Input: part model. Units: mm. Frame: model coordinates. A direction names the side the tool comes from. Give positions to 0.01 mm unless a question says otherwise; leave off trailing zeros. Loops run counter-clockwise (first coordinate to the right, second up) from the corner with the lowest first, then second, coordinate; pieces in that order, holes last. Notation, with made-up numbers: M -8.5,78 L 28.5,78 A31 cw 28.5,107 Z; hole C -11.5,89.5 d7. An arc over 180 degrees is marked long. Answer as a JSON object with one key per item and string values. Group by question number.
1) Section query C-C on y = 14.5. Return loops of the section in (x, z), plus the area to 3 significant figures.
2) Section query D-D on z = 1.5. Return loops of the section in (x, y).
3) Ray query, L1, parallel to X at y = 0, z = 8.5; L2, parallel to Y at x = 0, z = 9.25; L3, parallel to Y at x = -1, z = 3. Return the intervals inside material, ascending.
4) First-contact query: P1, Ø12, axis at y = 23, z = 7, coming from the -X side; P2, Ø8, axis at y = 26.5, z = 13.5, coming from the +X side; P3, Ø2.5, axis at x = -0.5, z = 5, coming from the +Y side; P4, Ø5, axis at x = 0.5, z = 17, coming from the -Y side. Flat tips, straight axial feed; report the tip coordinate or a pass-through.
5) Access query for faces 1 (the flat face through (-1.877, 3.143, 9.86)), 2 (the flat face through (-2.5, 24, 10)), 3 (the flat face through (0, 3.921, 5)), 4 (the flat face through (0, 43.921, 9.6)). Directions: +Z, -Z, +X, -X, +Y, -Y. A direction counts if a zero-diameter tool reaches every point of the face in a straight line with its end or side. Return the directions, or none.
6) Draft query along Z for faces 5 (the flat face through (2.5, 24, 10)), 6 (the cylindrical face through (-0.04, 40.91, 17.15)), 7 (the flat face through (0, 5, 2.5)). Return one class per face: +Z half, -Z half, draft (parallel to the pull), parting line (faces both ways), or undercut.
7) Section query B-B on z = 15. Return loops of the section in (x, y), plus the area to 3 significant figures.
8) Section query A-A on x = 1. Return loops of the section in (y, z).
from build123d import *

# Parameters (mm, degrees)
F1_DEPTH = 20
F3_DEPTH = 7.151
F4_R     = 10
F5_SIZE  = 5
F6_R     = 10


with BuildPart() as f1:
    # F0 (on Top) → F1 (new body)
    with BuildSketch(Plane.XY):
        with BuildLine():
            ThreePointArc((2.65, 0), (-0.9156644986, -2.4867767343), (-2.0172139819, 1.7185306955))
            Line((-2.0172139819, 1.7185306955), (-2.6488466474, 2.5070635361))
            Line((-2.6488466474, 2.5070635361), (-3.2804793129, 3.2955963767))
            ThreePointArc((-3.2804793129, 3.2955963767), (-1.7844146372, -4.2939916631), (4.65, 0))
            ThreePointArc((4.65, 0), (4.0772233199, 2.2357884515), (2.5, 3.920777984))
            ThreePointArc((2.5, 3.920777984), (1.3020910825, 4.4639734333), (0, 4.65))
            Line((0, 4.65), (0, 2.65))
            ThreePointArc((0, 2.65), (1.8738329701, 1.8738329701), (2.65, 0))
        make_face()
        with BuildLine():
            Line((0, 43.920777984), (0, 4.65))
            ThreePointArc((0, 4.65), (1.3020910825, 4.4639734333), (2.5, 3.920777984))
            Line((2.5, 3.920777984), (2.5, 43.920777984))
            Line((2.5, 43.920777984), (0, 43.920777984))
        make_face()
        with BuildLine():
            ThreePointArc((-1.236734669, 2.3437123028), (-0.6370488198, 2.572288631), (0, 2.65))
            Line((0, 2.65), (0, 4.65))
            ThreePointArc((0, 4.65), (-1.3020910825, 4.4639734333), (-2.5, 3.920777984))
            Line((-2.5, 3.920777984), (-1.8683673345, 3.1322451434))
            Line((-1.8683673345, 3.1322451434), (-1.236734669, 2.3437123028))
        make_face()
        with BuildLine():
            ThreePointArc((-2.5, 3.920777984), (-1.3020910825, 4.4639734333), (0, 4.65))
            Line((0, 4.65), (0, 43.920777984))
            Line((0, 43.920777984), (-2.5, 43.920777984))
            Line((-2.5, 43.920777984), (-2.5, 3.920777984))
        make_face()
    extrude(amount=F1_DEPTH)

    # F2 (on face) → F3 (cut, through all)
    with BuildSketch(Plane(origin=(-2.5, 0, 0), x_dir=(0, -1, 0), z_dir=(-1, 0, 0))):
        with BuildLine():
            Line((-33.920777984, 10), (-33.920777984, 12.25))
            ThreePointArc((-33.920777984, 12.25), (-35.5117682417, 11.5909902577), (-36.170777984, 10))
            Line((-36.170777984, 10), (-33.920777984, 10))
        make_face()
        with BuildLine():
            ThreePointArc((-36.170777984, 10), (-33.920777984, 7.75), (-31.670777984, 10))
            ThreePointArc((-31.670777984, 10), (-32.3297877264, 11.5909902577), (-33.920777984, 12.25))
            Line((-33.920777984, 12.25), (-33.920777984, 10))
            Line((-33.920777984, 10), (-36.170777984, 10))
        make_face()
        Polygon((-3.920777984, 17.5), (-5.420777984, 17.5), (-6.920777984, 17.5), (-6.920777984, 12.5), (-3.920777984, 12.5), align=None)
        Polygon((-6.920777984, 2.5), (-5.420777984, 2.5), (-3.920777984, 2.5), (-3.920777984, 7.5), (-6.920777984, 7.5), align=None)
    extrude(amount=-F3_DEPTH, mode=Mode.SUBTRACT)

    # F4
    f4_edges = [f1.edges().sort_by_distance(p)[0] for p in [
        (0, 43.920778, 20),
    ]]
    fillet(f4_edges, radius=F4_R)

    # F5
    f5_edges = [f1.edges().sort_by_distance(p)[0] for p in [
        (0, 43.920778, 0),
    ]]
    chamfer(f5_edges, length=F5_SIZE)

    # F6
    f6_edges = [f1.edges().sort_by_distance(p)[0] for p in [
        (0, 43.920778, 5),
    ]]
    fillet(f6_edges, radius=F6_R)


solid = f1.part
Output:
{
 "1": {"outline": "M -2.5,0 L 2.5,0 L 2.5,20 L -2.5,20 Z", "area": "100 mm^2"},
 "2": {"outline": "M -3.28,3.3 A4.65 ccw long 2.5,3.92 L 2.5,40.42 L -2.5,40.42 L -2.5,3.92 L -1.24,2.34 A2.65 cw long -2.02,1.72 Z"},
 "3": {"L1": "x = -4.65 to -2.65, 2.65 to 4.65", "L2": "y = -4.65 to -2.65, 2.65 to 31.8, 36.04 to 43.92", "L3": "y = -4.54 to -2.45, 2.45 to 3.92, 6.92 to 41.81"},
 "4": {"P1": "stops at x = -2.5", "P2": "stops at x = 2.5", "P3": "stops at y = 43.49", "P4": "stops at y = -4.65"},
 "5": {"face 1": "+Z, -Z", "face 2": "+Z, -Z, -X, +Y", "face 3": "+X, -X", "face 4": "+Z, -Z, +X, -X, +Y"},
 "6": {"face 5": "draft", "face 6": "+Z half", "face 7": "undercut"},
 "7": {"outline": "M -3.28,3.3 A4.65 ccw long 2.5,3.92 L -2.5,3.92 L -1.24,2.34 A2.65 cw long -2.02,1.72 Z; M -2.5,6.92 L 2.5,6.92 L 2.5,42.58 L -2.5,42.58 Z", "area": "220 mm^2"},
 "8": {"outline": "M -4.54,0 L -2.45,0 L -2.45,20 L -4.54,20 Z; M 2.45,0 L 38.92,0 L 40.99,2.07 A10 ccw 43.92,9.14 L 43.92,10 A10 ccw 33.92,20 L 2.45,20 Z; hole M 3.92,2.5 L 6.92,2.5 L 6.92,7.5 L 3.92,7.5 Z; hole M 3.92,12.5 L 6.92,12.5 L 6.92,17.5 L 3.92,17.5 Z; hole C 33.92,10 d4.5"}
}
